Answer from the drawing. Dimensions are ordinates in mm from the lowest x, y and z of the part. Coordinates: 2 decimals unless noted, no trailing zeros. Write each loop counter-clockwise with the first axis right and the second up, starting at its lowest first coordinate (ties: lowest second). Pieces come first, ordered by that corner, then holes. Notation, with made-up numbers: (34.25, -39) -> (67.25, -39) arc R31 ccw to (67.25, -1) -> close; hole circle Ø10 at (74, 12). An arc over 180 degrees is marked (long way). Use CSV: the item, a comma, the result in double quotes.
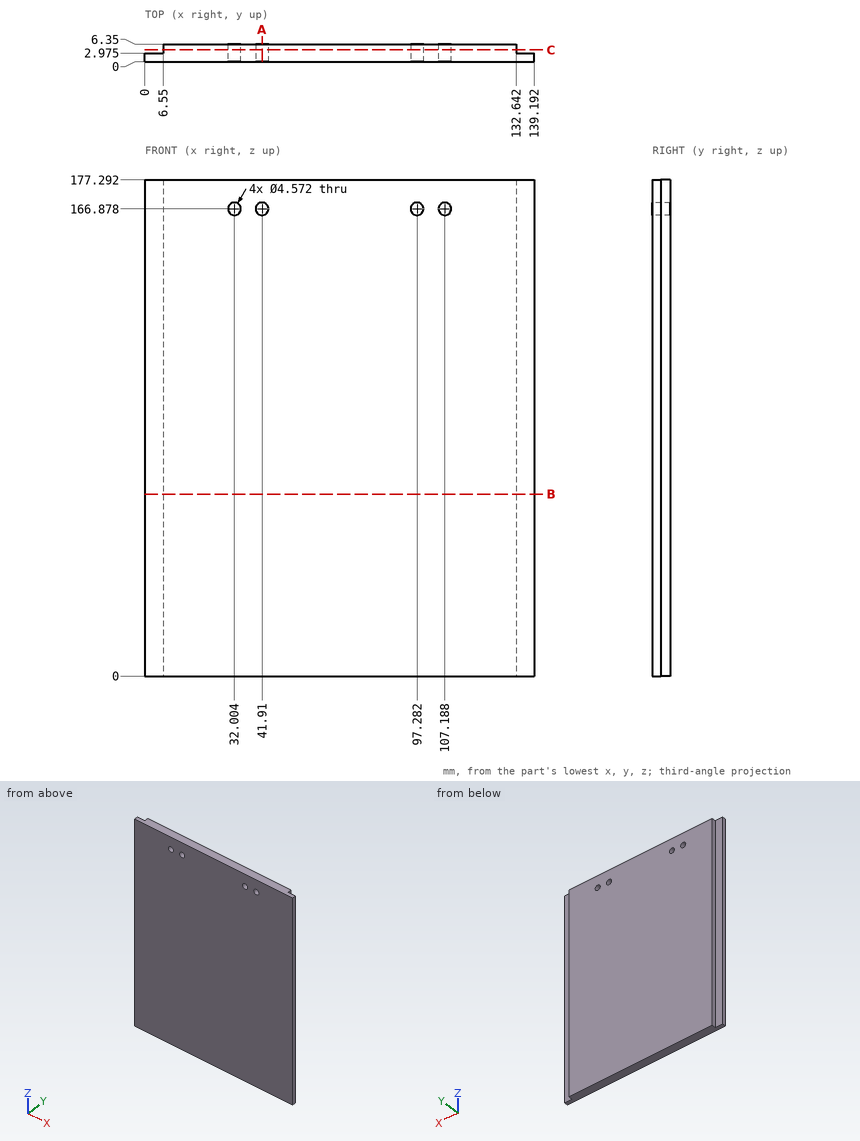
1. A cutting plane is placed at A-A (x = 41.91). Give the vertices of the cut face in (y, z).
Solutions:
outline,"(0, 0) -> (6.35, 0) -> (6.35, 164.59) -> (0, 164.59) -> close; (0, 169.16) -> (6.35, 169.16) -> (6.35, 177.29) -> (0, 177.29) -> close"
2. A cutting plane is placed at B-B (z = 65). Give the vertices of the cut face in (x, y) (3 decimals).
Solutions:
outline,"(0, 0) -> (139.192, 0) -> (139.192, 2.975) -> (132.642, 2.975) -> (132.642, 6.35) -> (6.55, 6.35) -> (6.55, 2.975) -> (0, 2.975) -> close"
3. Each of these flat-tipped pins is pushed along its axis until it touches: pin 1 Ø1.7 at (y, z) = (5, 94) entering from +X; pin 2 Ø1 at (y, z) = (4.5, 126) entering from -X; pin 3 Ø3.5 at (x, z) = (2, 129) entering from +Y (3 decimals). Where does it stop, or does it pass through?
Solutions:
pin 1,"stops at x = 132.64"
pin 2,"stops at x = 6.55"
pin 3,"stops at y = 2.975"
4. A cutting plane is placed at C-C (y = 4.25). Give the vertices of the cut face in (x, z).
Solutions:
outline,"(6.55, 0) -> (132.64, 0) -> (132.64, 177.29) -> (6.55, 177.29) -> close; hole circle Ø4.57 at (32, 166.88); hole circle Ø4.57 at (41.91, 166.88); hole circle Ø4.57 at (97.28, 166.88); hole circle Ø4.57 at (107.19, 166.88)"
5. Find the intervals of material crossed by line 1 along Z through (x, y) = (41.91, 2.75); line 2 along X through (y, z) = (6, 31.5); line 3 along Z through (x, y) = (40.5, 5.5), in increasing order.
Solutions:
line 1,"z = 0 to 164.59, 169.16 to 177.29"
line 2,"x = 6.55 to 132.64"
line 3,"z = 0 to 165.08, 168.68 to 177.29"
